Can you work these out from the model? Positions are in its coordinate system, mm. Face numbers are marked on the shaded views. A direction names the side the tool comes from. Give positions to 0.01 mm unless a question says otherwise; leave off trailing zeros. Write each loop counter-clockwise with the first axis right and the second up, starting at its lowest first coordinate (ties: lowest second). Pieces come first, ordered by that corner, then holes. Notation, with made-up numbers: (-22, 55.5) - (-10, 55.5) arc R20 cw to (-10, 84.5) - close; hole circle Ø2 at (83.5, 55). An arc over 180 degrees is marked (long way). Use a Markdown table: item, result. Add a question column.
Autodesk Inventor part; units mm, degrees
ref_plane "YZ Plane" through (0, 0, 0) normal (1, 0, 0) x (0, 1, 0)
ref_plane "XZ Plane" through (0, 0, 0) normal (0, 1, 0) x (-1, 0, 0)
ref_plane "XY Plane" through (0, 0, 0) normal (0, 0, 1) x (1, 0, 0)
sketch "Sketch1" plane through (0, 0, 0) normal (0, 1, 0) x (-1, 0, 0)
  circle A0 centre (0, 0) radius 8.5
  dimension "d0" = 17
extrude "Extrusion1" add sketch "Sketch1" along normal blind 40
sketch "Sketch2" plane through (0, 40, 0) normal (0, 1, 0) x (1, 0, 0)
  circle A0 centre (0, 0) radius 8.5
  line L0 (0, 0) -> (0, 4.25)
  line L1 (0, 4.25) -> (-2, 4.25)
  line L2 (-2, 4.25) -> (-2, -4.25)
  line L3 (-2, -4.25) -> (2, -4.25)
  line L4 (2, -4.25) -> (2, 4.25)
  line L5 (2, 4.25) -> (0, 4.25)
  dimension "d3" = 4.25
  dimension "d4" = 2
  dimension "d5" = 8.5
  dimension "d6" = 4
extrude "Extrusion2" add sketch "Sketch2" along normal blind 10.6 contours L5 L4 L3 L2 L1
fillet "Fillet1" radius 3.5 2 edges at (0, 50.6, 4.25) (0, 50.6, -4.25)
sketch "Sketch3" plane through (2, 40, 4.25) normal (1, 0, 0) x (0, 0, -1)
  circle A0 centre (4.25, 6.45) radius 2.75
  line L0 (3.5, 10.6) -> (5, 10.6)
  point P0 (4.25, -40)
  dimension "d11" = 5.5
  dimension "d26" = 4.15
extrude "Extrusion3" cut sketch "Sketch3" against normal blind 10.5
sketch "Sketch4" plane through (0, 0, 0) normal (0, -1, 0) x (1, 0, 0)
  circle A0 centre (0, 0) radius 8.5
  line L0 (0, 0) -> (0, 4.5)
  line L1 (0, 4.5) -> (-3, 4.5)
  line L2 (-3, 4.5) -> (-3, -4.5)
  line L3 (-3, -4.5) -> (3, -4.5)
  line L4 (3, -4.5) -> (3, 4.5)
  line L5 (3, 4.5) -> (0, 4.5)
  dimension "d14" = 4.5
  dimension "d15" = 3
  dimension "d16" = 9
  dimension "d17" = 6
extrude "Extrusion4" add sketch "Sketch4" along normal blind 16.6 contours L5 L4 L3 L2 L1
fillet "Fillet2" radius 4 2 edges at (0, -16.6, -4.5) (0, -16.6, 4.5)
sketch "Sketch5" plane through (3, 0, 4.5) normal (1, 0, 0) x (0, 0, -1)
  circle A0 centre (4.5, -12.7) radius 1.5
  line L0 (4, -16.6) -> (5, -16.6)
  point P0 (4.5, 0)
  dimension "d22" = 3
  dimension "d27" = 3.9
extrude "Extrusion5" cut sketch "Sketch5" against normal blind 16.5
equation "\"d15\" = 0.5 * d17"
properties part number "pruzina"
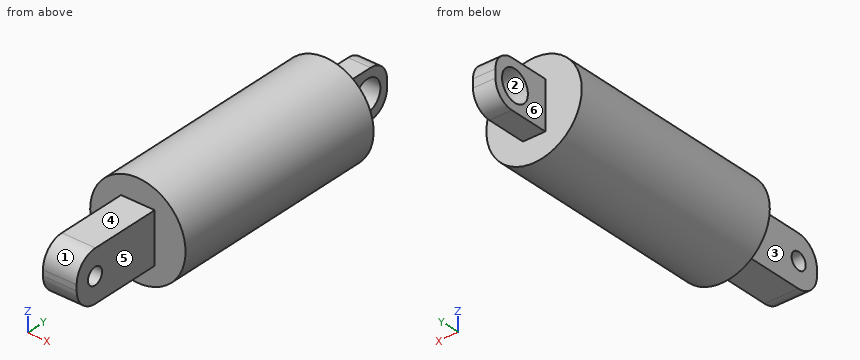
Q1. Suppose I cut it at C-C (y = 39). Please give me the cut outline in (x, z).
Q2. I'm going to push flat-ended pins straight in: P1, Ø5, axis at x = -3.5, z = -1.5, coming from the -Y side; P2, Ø2, axis at x = 1.5, y = -7, coming from the -Z side; P3, Ø4, axis at x = -6.5, y = 0.5, coming from the -Z side; P4, Ø2, axis at x = -3.5, y = 31, coming from the -Z side. Where does each tip first touch, or does it pass through?
Q3. Suppose I cut it at A-A (y = 46.45). Please give me the cut outline in (x, z).
Q4. If I drill on probe 1 along Y at (x, z) = (-1.45, 0); probe 2 along Y at (x, z) = (0.25, 0.5); probe 3 along X at (y, z) = (28, -0.5), over which ranges is the centre line in solid material (lowest first)? Write a range as [from, to].
Q5. Suppose I cut it at D-D (z = -7.25). Please give me the cut outline in (x, y).
Q6. If we mould it in two halves opening along Z, with no side actions, what happens to the marked faces 1, 2 and 3? For each: released by +Z, released by -Z, zero draft, split by the parting line, or undercut.
Q7. On a 3-axis mill with a long thin cutter (end or side, diameter ignored), from which of +Z, -Z, +X, -X, +Y, -Y can I reach the whole of each face in a straight line? I mean the marked faces 4, 5 and 6. Say none if no direction works.
Q8. Suppose I cut it at B-B (x = 0). Please give me the cut outline in (y, z).
Derived:
| question | item | result |
|---|---|---|
| 1 | outline | circle Ø17 at (0, 0) |
| 2 | P1 | y = -16.6 |
| 2 | P2 | z = -4.5 |
| 2 | P3 | z = -7.21 |
| 2 | P4 | z = -8.12 |
| 3 | outline | (-2, -4.25) - (2, -4.25) - (2, -2.75) - (-2, -2.75) - close; (-2, 2.75) - (2, 2.75) - (2, 4.25) - (-2, 4.25) - close |
| 4 | probe 1 | [-16.6, -14.2], [-11.2, 43.7], [49.2, 50.6] |
| 4 | probe 2 | [-16.6, -14.11], [-11.29, 43.75], [49.15, 50.6] |
| 4 | probe 3 | [-8.49, 8.49] |
| 5 | outline | (-4.44, 0) - (4.44, 0) - (4.44, 40) - (-4.44, 40) - close |
| 6 | face 1 | released by +Z |
| 6 | face 2 | undercut |
| 6 | face 3 | zero draft |
| 7 | face 4 | +Z, +X, -X, -Y |
| 7 | face 5 | +Z, -Z, +X, -Y |
| 7 | face 6 | +Z, -Z, -X, +Y |
| 8 | outline | (-16.6, -0.5) arc R4 ccw to (-12.6, -4.5) - (0, -4.5) - (0, -8.5) - (40, -8.5) - (40, -4.25) - (47.1, -4.25) arc R3.5 ccw to (50.6, -0.75) - (50.6, 0.75) arc R3.5 ccw to (47.1, 4.25) - (40, 4.25) - (40, 8.5) - (0, 8.5) - (0, 4.5) - (-12.6, 4.5) arc R4 ccw to (-16.6, 0.5) - close; hole circle Ø3 at (-12.7, 0); hole circle Ø5.5 at (46.45, 0) |
